Here's how the part is built. I have some questions about the finished solid (model axes, mm). Face numbers are marked on the shaded views. A direction names the side the tool comes from. Coordinates: 2 decimals unless noted, no trailing zeros. Write each loop counter-clockwise with the first axis right and the second up, starting at its lowest first coordinate (ties: lowest second). Pieces come first, ordered by that corner, then holes. Notation, with made-up numbers: (-31, 13) -> (-7, 13) arc R28 ccw to (-7, 51) -> close; hole circle Ø8 at (-24, -22.75). An arc over 180 degrees is marked (long way). Use CSV: the item, a comma, the result in double quotes. Start each with the question number.
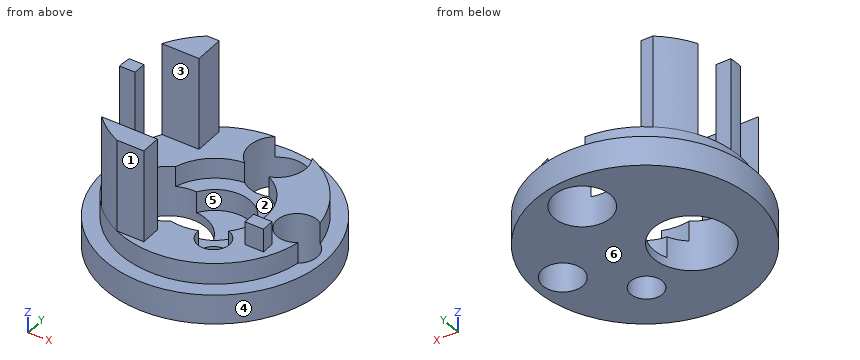
```python
from build123d import *

# Parameters (mm, degrees)
F2_R     = 21.6962130455
F2_R_2   = 17.1617704493
F2_R_3   = 40.953196501
F2_R_4   = 30.4988959279
F3_DEPTH = 1000
F5_DEPTH = 100
F6_W     = 19.7006091475
F6_H     = 13.662148267
F7_DEPTH = 25


# Not quite as in the source:
# - after a boolean that leaves OpenCascade's solid faulty, fix() repairs it


with BuildPart() as f1:
    # F0 (on Front) → F1 (revolve)
    with BuildSketch(Plane.XZ):
        Polygon((0, 9.6338680014), (0, 0), (118.4682399035, 0), (118.4682399035, 31.7357704043), (102.0300611854, 31.7357704043), (102.0300611854, 54.4380694628), (54.9828708172, 54.4380694628), (54.9828708172, 32.5937792659), (37.9778593779, 32.5937792659), (37.9778593779, 9.6338680014), align=None)
    revolve(axis=Axis((0, 0, 4.8169340007), (0, 0, -1)))

    # F2 (on face) → F3 (cut)
    with BuildSketch(Plane(origin=(0, 0, 0), x_dir=(1, 0, 0), z_dir=(0, 0, -1))):
        with Locations((87.8278240561, 0)):
            Circle(F2_R)
        with Locations((34.7668491304, 54.0037713945)):
            Circle(F2_R_2)
        with Locations((-35.4811474681, 21.4303005487)):
            Circle(F2_R_3)
        with Locations((14.2781008035, -78.1974196434)):
            Circle(F2_R_4)
    extrude(amount=-F3_DEPTH, mode=Mode.SUBTRACT)

    # F4 (on face) → F5 (join)
    with BuildSketch(Plane.XY.offset(54.4380694628)):
        with BuildLine():
            Line((-49.8583316803, 48.6504090547), (-49.8583316803, 80.5302113295))
            Line((-49.8583316803, 80.5302113295), (-62.6499676674, 80.5302113295))
            ThreePointArc((-62.6499676674, 80.5302113295), (-77.8171679529, 65.9895579412), (-89.684285604, 48.6504090547))
            Line((-89.684285604, 48.6504090547), (-49.8583316803, 48.6504090547))
        make_face()
        with BuildLine():
            Line((-85.3846818209, 13.8626152044), (-101.0839318843, 13.8626152044))
            ThreePointArc((-101.0839318843, 13.8626152044), (-101.7932540508, 6.9474322767), (-102.0300611854, 0))
            Line((-102.0300611854, 0), (-85.3846818209, 0))
            Line((-85.3846818209, 0), (-85.3846818209, 13.8626152044))
        make_face()
        with BuildLine():
            Line((-13.3902756497, -71.5824663639), (-72.7054598689, -71.5824663639))
            ThreePointArc((-72.7054598689, -71.5824663639), (-58.4249180154, -83.6460539439), (-42.1830749936, -92.9016768932))
            Line((-42.1830749936, -92.9016768932), (-13.3902756497, -92.9016768932))
            Line((-13.3902756497, -92.9016768932), (-13.3902756497, -71.5824663639))
        make_face()
    extrude(amount=F5_DEPTH)

    add(f1.part.fix(), mode=Mode.REPLACE)

    # F6 (on face) → F7 (join)
    with BuildSketch(Plane.XY.offset(54.4380694628)):
        with Locations((73.1044746935, -39.3697526306)):
            Rectangle(F6_W, F6_H)
    extrude(amount=F7_DEPTH)


solid = f1.part
```
Item 1: Which directions (+Z, -Z, +X, -X, +Y, -Y) give clear straight access to the entire face, cutting with the end or side of a thin tool? Please do the marked faces 1, 2 and 3.
Item 2: I want a section at C-C on z = 58.5. Please give me the cut outline in (x, y).
Item 3: I want a section at D-D on y = 65. Please give me the cut outline in (x, z), then the cut area to 3 significant figures.
Item 4: I want a section at B-B on x = -46. Please give me the cut outline in (y, z), then the cut area to 3 significant figures.
Item 5: I want a section at A-A on z = 131. Please give me the cut outline in (x, y), then the cut area to 3 significant figures.
Item 6: Thinking about a two-plate mould opening in X: for the marked faces 4, 5 and 6, which applies, +X half, -X half, draft (parallel to the pull), parting line (faces both ways), or undercut?
Item 7: I'm going to push flat-ended pins straight in: pin 1 (12 mm diameter, centred on y = -10.5, z = 113.5, fed in from +X); pin 2 (17 mm diameter, centred on y = -84, z = 116, fed in from +X); pin 3 (8 mm diameter, centred on x = -82, y = -82, fed in from -Z); pin 4 (7 mm diameter, centred on x = 71.5, y = -36, fed in from +Z). Where does each tip first touch, or does it pass through?
Item 8: If I drill on line 1 along Y through (x, z) = (0, 27.5); line 2 along Y through (x, z) = (-8.5, 15); line 3 along Z through (x, y) = (-38, -101), over which ranges is the centre line in solid material (lowest first)?
Geometry says:
1,face 1,"+Z, +X, -X, -Y"
1,face 2,"+Z"
1,face 3,"+Z, +X, -X"
2,outline,"(-102.03, 0) -> (-85.38, 0) -> (-85.38, 13.86) -> (-101.08, 13.86) arc R102.03 ccw to start; (-89.68, 48.65) -> (-49.86, 48.65) -> (-49.86, 80.53) -> (-62.65, 80.53) arc R102.03 ccw to start; (-72.71, -71.58) arc R102.03 ccw to (-42.18, -92.9) -> (-13.39, -92.9) -> (-13.39, -71.58) -> close; (63.25, -46.2) -> (82.95, -46.2) -> (82.95, -32.54) -> (63.25, -32.54) -> close"
3,outline,"(-99.04, 0) -> (-13.22, 0) -> (-13.22, 54.44) -> (-49.86, 54.44) -> (-49.86, 154.44) -> (-78.65, 154.44) -> (-78.65, 31.74) -> (-99.04, 31.74) -> close; (41.77, 0) -> (99.04, 0) -> (99.04, 31.74) -> (78.65, 31.74) -> (78.65, 54.44) -> (41.77, 54.44) -> close"
3,area,"9,740 mm2"
4,outline,"(-109.17, 0) -> (-61.01, 0) -> (-61.01, 54.44) -> (-71.58, 54.44) -> (-71.58, 154.44) -> (-91.07, 154.44) -> (-91.07, 31.74) -> (-109.17, 31.74) -> close; (18.15, 0) -> (109.17, 0) -> (109.17, 31.74) -> (91.07, 31.74) -> (91.07, 54.44) -> (30.12, 54.44) -> (30.12, 32.59) -> (18.15, 32.59) -> close"
4,area,"8,440 mm2"
5,outline,"(-102.03, 0) -> (-85.38, 0) -> (-85.38, 13.86) -> (-101.08, 13.86) arc R102.03 ccw to start; (-89.68, 48.65) -> (-49.86, 48.65) -> (-49.86, 80.53) -> (-62.65, 80.53) arc R102.03 ccw to start; (-72.71, -71.58) arc R102.03 ccw to (-42.18, -92.9) -> (-13.39, -92.9) -> (-13.39, -71.58) -> close"
5,area,"2,110 mm2"
6,face 4,"parting line"
6,face 5,"undercut"
6,face 6,"draft"
7,pin 1,"through"
7,pin 2,"x = -13.39"
7,pin 3,"z = 0"
7,pin 4,"z = 79.44"
8,line 1,"-118.47 to -41.88, 37.98 to 51.25, 105.15 to 118.47"
8,line 2,"-118.16 to -52.24, 37.01 to 57.92, 98.48 to 118.16"
8,line 3,"0 to 31.74"
